from build123d import *

# Parameters (mm, degrees)
F0_W     = 148
F0_H     = 14.2765273312
F1_DEPTH = 133.35
F2_W     = 18
F2_H     = 12.7
F3_DEPTH = 14.2775273312


with BuildPart() as f1:
    # F0 (on Top) → F1 (new body, symmetric)
    with BuildSketch(Plane.XY):
        with Locations((-106.1730651801, 2.7383093525)):
            Rectangle(F0_W, F0_H)
    extrude(amount=F1_DEPTH, both=True)

    # F2 (on face) → F3 (cut, through all)
    with BuildSketch(Plane.XZ.offset(4.3999543131)):
        with Locations((-390.5, -12.7)):
            Rectangle(F2_W, F2_H)
        with Locations((-390.5, -38.1)):
            Rectangle(F2_W, F2_H)
        with Locations((-390.5, -63.5)):
            Rectangle(F2_W, F2_H)
        with Locations((-390.5, -88.9)):
            Rectangle(F2_W, F2_H)
        with Locations((-390.5, -114.3)):
            Rectangle(F2_W, F2_H)
        Polygon((-265, 113.35), (-265, 120.65), (-283, 120.65), (-283, 107.95), (-265, 107.95), align=None)
        with Locations((-274, 12.7)):
            Rectangle(F2_W, F2_H)
        Polygon((-265, 44.45), (-283, 44.45), (-283, 31.75), (-265, 31.75), (-265, 33.35), align=None)
        with Locations((-274, 63.5)):
            Rectangle(F2_W, F2_H)
        with Locations((-274, 88.9)):
            Rectangle(F2_W, F2_H)
        with Locations((-171.1730651801, -114.3)):
            Rectangle(F2_W, F2_H)
        Polygon((-162.1730651801, -95.25), (-162.1730651801, -82.55), (-180.1730651801, -82.55), (-180.1730651801, -95.25), (-163.5, -95.25), align=None)
        with Locations((-171.1730651801, -63.5)):
            Rectangle(F2_W, F2_H)
        with Locations((-171.1730651801, -38.1)):
            Rectangle(F2_W, F2_H)
        with Locations((-171.1730651801, -12.7)):
            Rectangle(F2_W, F2_H)
        with Locations((-171.1730651801, 12.7)):
            Rectangle(F2_W, F2_H)
        with Locations((-171.1730651801, 38.1)):
            Rectangle(F2_W, F2_H)
        with Locations((-171.1730651801, 63.5)):
            Rectangle(F2_W, F2_H)
        Polygon((-162.1730651801, 82.55), (-162.1730651801, 95.25), (-163.5, 95.25), (-180.1730651801, 95.25), (-180.1730651801, 82.55), align=None)
        with Locations((-171.1730651801, 114.3)):
            Rectangle(F2_W, F2_H)
    extrude(amount=-F3_DEPTH, mode=Mode.SUBTRACT)


solid = f1.part
Can you work these out from the model? Positions are in its coordinate system, mm. A direction names the side the tool comes from. Round coordinates to 2 decimals unless told otherwise and drop trailing zeros. Loops run counter-clockwise (first coordinate to the right, second up) from the corner with the lowest first, then second, coordinate; pieces in that order, holes last. Notation, with made-up numbers: (8, 84.25) - (59, 84.25) arc R22 cw to (59, 114.25) - close; hole circle Ø10 at (32.5, 56.25). An arc over 180 degrees is marked (long way). Answer in a Markdown table with one row per item. Add a question column.
Q1. I want a section at A-A on x = -165.5. Count the separate pieces of the cut face and the enclosed holes in it, and give its area (3 significant figures).
Q2. I want a section at B-B on z = -63. List the corners of the cut face in (x, y) for me, and give its area (3 significant figures).
Q3. We'd pull the mould along Z, two halves only. Please class faces 1 (the flat face through (-180.173, 3, 76)), 2 (the flat face through (-162.173, 3, -64)), 3 (the flat face through (-171, 3, -6.35)): pulls with the +Z half, pulls with the -Z half, needs draft (parallel to the pull), parting line crosses it, or undercut.
Q4. I need wall thicknesses on L1, parallel to X at y = -0.5, z = -14. Which ranges of the line are inside material? Lowest first, please.
Q5. Which directions (+Z, -Z, +X, -X, +Y, -Y) give clear straight access to the entire face, cutting with the end or side of a thin tool? Please do faces 4 (the flat face through (-171, 3, -31.75)), 5 (the flat face through (-32.173, 3, 2)).
A:
| question | item | result |
|---|---|---|
| 1 | separate pieces | 11 |
| 1 | enclosed holes | 0 |
| 1 | area | 1,990 mm^2 |
| 2 | outline | (-162.17, -4.4) - (-32.17, -4.4) - (-32.17, 9.88) - (-162.17, 9.88) - close |
| 2 | area | 1,860 mm^2 |
| 3 | face 1 | needs draft |
| 3 | face 2 | undercut |
| 3 | face 3 | undercut |
| 4 | L1 | -162.17 to -32.17 |
| 5 | face 4 | -X, +Y, -Y |
| 5 | face 5 | +Z, -Z, +X, +Y, -Y |
